Verification items for the finished model (mm, model axes). A direction names the side the tool comes from. Coordinates: 2 decimals unless noted, no trailing zeros. Write each loop counter-clockwise with the first axis right and the second up, starting at its lowest first coordinate (ties: lowest second). Pieces come first, ordered by that corner, then holes. Notation, with made-up numbers: M -20,-5 L -11,-5 A25 cw -11,10 Z; hole C 16.25,84 d7. An arc over 180 degrees is marked long. Answer in a Markdown table with one row per item.
from build123d import *

# Parameters (mm, degrees)
BOX_W         = 13
BOX_H         = 10
BOX_DEPTH     = 8
SKETCH_R      = 23
PAD_DEPTH     = 1
SKETCH001_R   = 23
SKETCH001_R_2 = 21.6
PAD001_DEPTH  = 25


with BuildPart() as usb:
    # Box → Box (new body)
    with BuildSketch(Plane(origin=(-6.5, 16, 1), x_dir=(1, 0, 0), z_dir=(0, 0, 1))):
        with Locations((6.5, 5)):
            Rectangle(BOX_W, BOX_H)
    extrude(amount=BOX_DEPTH)


with BuildPart() as cut:
    # Sketch → Pad (new body)
    with BuildSketch(Plane.XY):
        Circle(SKETCH_R)
    extrude(amount=PAD_DEPTH)

    # Sketch001 (on Face3 of Pad) → Pad001 (join)
    with BuildSketch(Plane.XY.offset(1)):
        Circle(SKETCH001_R)
        Circle(SKETCH001_R_2, mode=Mode.SUBTRACT)
    extrude(amount=PAD001_DEPTH)

    # Cut: cut USB
    add(usb.part, mode=Mode.SUBTRACT)


solid = cut.part
1) Sectioned sample at D-D (x = 9.5). Record the cut outline in (y, z), then the cut area to 3 significant figures.
Response values:
| item | result |
|---|---|
| outline | M -20.95,0 L 20.95,0 L 20.95,26 L 19.4,26 L 19.4,1 L -19.4,1 L -19.4,26 L -20.95,26 Z |
| area | 119 mm² |
2) Sectioned sample at C-C (z = 19.5). Record the cut outline in (x, y).
Response values:
| item | result |
|---|---|
| outline | C 0,0 d46; hole C 0,0 d43.2 |
3) Sectioned sample at B-B (y = 0). Record the cut outline in (x, z), then the cut area to 3 significant figures.
Response values:
| item | result |
|---|---|
| outline | M -23,0 L 23,0 L 23,26 L 21.6,26 L 21.6,1 L -21.6,1 L -21.6,26 L -23,26 Z |
| area | 116 mm² |
4) Sectioned sample at A-A (x = 0). Record the cut outline in (y, z).
Response values:
| item | result |
|---|---|
| outline | M -23,0 L 23,0 L 23,1 L -21.6,1 L -21.6,26 L -23,26 Z; M 21.6,9 L 23,9 L 23,26 L 21.6,26 Z |
5) Thickness scan on L1, parallel to Y at x = 0, z = 16; L2, parallel to Z at x = -6, y = -4.5; L3, parallel to Y at x = 6, z = 10.75. Record the ranges inside material, lowest first. Write a range as [from, to].
Response values:
| item | result |
|---|---|
| L1 | y = [-23, -21.6], [21.6, 23] |
| L2 | z = [0, 1] |
| L3 | y = [-22.2, -20.75], [20.75, 22.2] |
6) Depth check by flat-ended pin: pin 1 (8 mm diameter, centred on x = 14, y = -6, fed in from -Z); pin 2 (4 mm diameter, centred on y = -9, z = 16.5, fed in from -X); pin 3 (12 mm diameter, centred on x = 17, z = 19.5, fed in from +Y); pin 4 (4 mm diameter, centred on x = -17.5, z = 16.5, fed in from +Y). Enter the tip coordinate at first touch or a pass-through.
Response values:
| item | result |
|---|---|
| pin 1 | stops at z = 0 |
| pin 2 | stops at x = -21.91 |
| pin 3 | stops at y = 20.2 |
| pin 4 | stops at y = 16.99 |
7) Release check for a two-part mould opening along Z. For faces 1 (the face through (0, 0, 0)), 2 (the face through (6.5, 21, 5)), 3 (the face through (7, 21, 26)) record: +Z half, -Z half, draft (parallel to the pull), parting line (faces both ways), or undercut.
Response values:
| item | result |
|---|---|
| face 1 | -Z half |
| face 2 | undercut |
| face 3 | +Z half |
8) Tool access check on faces 4 (the face through (-4.682, -21.086, 13.325)), 5 (the face through (0, 22, 9)), 6 (the face through (-4.986, -22.453, 12.818)). Record the directions out of +Z, -Z, +X, -X, +Y, -Y that give a thin tool (end or side, any length) a straight path to the whole face; none if there is none.
Response values:
| item | result |
|---|---|
| face 4 | +Z |
| face 5 | +Y |
| face 6 | +Z, -Z |
